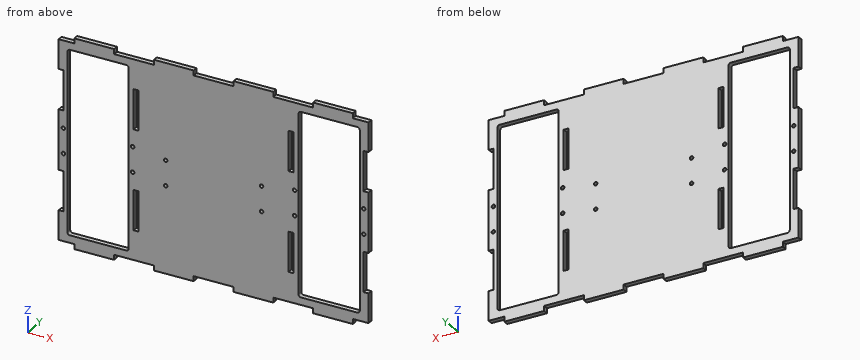
from build123d import *

# Parameters (mm, degrees)
SKETCH5_W             = 395.4
SKETCH5_H             = 265.4
BOSS_EXTRUDE3_DEPTH   = 6.35
SKETCH6_W             = 78.175
SKETCH6_H             = 243.175
SKETCH6_W_2           = 75
SKETCH6_H_2           = 240
CUT_EXTRUDE1_DEPTH    = 6.35
F_4_0MM_DOWEL_HOLE1_D = 4.5
SKETCH10_W            = 6.35
SKETCH10_H            = 50.8
SKETCH10_W_2          = 50.8
SKETCH10_H_2          = 6.35
CUT_EXTRUDE2_DEPTH    = 6.35
SKETCH11_W            = 50.8
SKETCH11_H            = 6.35
CUT_EXTRUDE3_DEPTH    = 6.35
SKETCH12_W            = 78.175
SKETCH12_H            = 4.7625
BOSS_EXTRUDE4_DEPTH   = 6.35
FILLET1_R             = 3.175


with BuildPart() as part:
    # Sketch5 → Boss-Extrude3 (new body)
    with BuildSketch(Plane(origin=(0, 0, 0), x_dir=(1, 0, 0), z_dir=(0, 1, 0))):
        Rectangle(SKETCH5_W, SKETCH5_H)
    extrude(amount=BOSS_EXTRUDE3_DEPTH)

    # Sketch6 → Cut-Extrude1 (cut)
    # profile 1 of 4: a face of its own
    with BuildSketch(Plane(origin=(0, 6.35, 0), x_dir=(1, 0, 0), z_dir=(0, 1, 0))):
        with Locations((147.5, 0)):
            Rectangle(SKETCH6_W, SKETCH6_H)
        with Locations((147.5, 0)):
            Rectangle(SKETCH6_W_2, SKETCH6_H_2, mode=Mode.SUBTRACT)
    # profile 2 of 4: a face of its own
    with BuildSketch(Plane(origin=(0, 6.35, 0), x_dir=(1, 0, 0), z_dir=(0, 1, 0))):
        with Locations((147.5, 0)):
            Rectangle(SKETCH6_W_2, SKETCH6_H_2)
    # profile 3 of 4: a face of its own
    with BuildSketch(Plane(origin=(0, 6.35, 0), x_dir=(1, 0, 0), z_dir=(0, 1, 0))):
        with Locations((-147.5, 0)):
            Rectangle(SKETCH6_W, SKETCH6_H)
        with Locations((-147.5, 0)):
            Rectangle(SKETCH6_W_2, SKETCH6_H_2, mode=Mode.SUBTRACT)
    # profile 4 of 4: a face of its own
    with BuildSketch(Plane(origin=(0, 6.35, 0), x_dir=(1, 0, 0), z_dir=(0, 1, 0))):
        with Locations((-147.5, 0)):
            Rectangle(SKETCH6_W_2, SKETCH6_H_2)
    extrude(amount=-CUT_EXTRUDE1_DEPTH, mode=Mode.SUBTRACT)

    # Ø4.0mm Dowel Hole1 (through all)
    with Locations(Plane(origin=(0, 6.35, 0), x_dir=(1, 0, 0), z_dir=(0, 1, 0))):
        with Locations((191.675, -16), (191.675, 16), (103.325, -16), (103.325, 16), (-191.675, -16), (-191.675, 16), (-103.325, -16), (-103.325, 16), (-61.175, -10), (-61.175, 22), (61.175, 22), (61.175, -10)):
            Hole(F_4_0MM_DOWEL_HOLE1_D / 2)

    # Sketch10 → Cut-Extrude2 (cut)
    with BuildSketch(Plane.XZ):
        with Locations((98.8875, -63.5)):
            Rectangle(SKETCH10_W, SKETCH10_H)
        with Locations((98.8875, 63.5)):
            Rectangle(SKETCH10_W, SKETCH10_H)
        with Locations((-98.8875, 63.5)):
            Rectangle(SKETCH10_W, SKETCH10_H)
        with Locations((-98.8875, -63.5)):
            Rectangle(SKETCH10_W, SKETCH10_H)
        Polygon((197.7, 132.7), (177.8, 132.7), (177.8, 126.35), (191.35, 126.35), (197.7, 126.35), align=None)
        Polygon((127, 132.7), (76.2, 132.7), (76.2, 126.35), (95.7125, 126.35), (102.0625, 126.35), (108.4125, 126.35), (127, 126.35), align=None)
        with Locations((0, 129.525)):
            Rectangle(SKETCH10_W_2, SKETCH10_H_2)
        Polygon((-127, 132.7), (-127, 126.35), (-108.4125, 126.35), (-102.0625, 126.35), (-95.7125, 126.35), (-76.2, 126.35), (-76.2, 132.7), align=None)
        Polygon((-197.7, 126.35), (-191.35, 126.35), (-177.8, 126.35), (-177.8, 132.7), (-197.7, 132.7), align=None)
        Polygon((-177.8, -126.35), (-191.35, -126.35), (-197.7, -126.35), (-197.7, -132.7), (-177.8, -132.7), align=None)
        Polygon((-108.4125, -126.35), (-127, -126.35), (-127, -132.7), (-76.2, -132.7), (-76.2, -126.35), (-95.7125, -126.35), (-102.0625, -126.35), align=None)
        with Locations((0, -129.525)):
            Rectangle(SKETCH10_W_2, SKETCH10_H_2)
        Polygon((76.2, -126.35), (76.2, -132.7), (127, -132.7), (127, -126.35), (108.4125, -126.35), (102.0625, -126.35), (95.7125, -126.35), align=None)
        Polygon((177.8, -126.35), (177.8, -132.7), (197.7, -132.7), (197.7, -126.35), (191.35, -126.35), align=None)
    extrude(amount=-CUT_EXTRUDE2_DEPTH, mode=Mode.SUBTRACT)

    # Sketch11 → Cut-Extrude3 (cut)
    with BuildSketch(Plane(origin=(197.7, 0, 0), x_dir=(0, 0, -1), z_dir=(1, 0, 0))):
        with Locations((-63.5, 3.175)):
            Rectangle(SKETCH11_W, SKETCH11_H)
        with Locations((63.5, 3.175)):
            Rectangle(SKETCH11_W, SKETCH11_H)
    cut_extrude3 = extrude(amount=-CUT_EXTRUDE3_DEPTH, mode=Mode.SUBTRACT)

    # Mirror1: Cut-Extrude3 across plane
    add(cut_extrude3.mirror(Plane(origin=(0, 0, 0), x_dir=(0, 0, 1), z_dir=(1, 0, 0))), mode=Mode.SUBTRACT)

    # Sketch12 → Boss-Extrude4 (add)
    with BuildSketch(Plane.XZ):
        with Locations((147.5, -119.20625)):
            Rectangle(SKETCH12_W, SKETCH12_H)
        with Locations((147.5, 119.20625)):
            Rectangle(SKETCH12_W, SKETCH12_H)
        with Locations((-147.5, 119.20625)):
            Rectangle(SKETCH12_W, SKETCH12_H)
        with Locations((-147.5, -119.20625)):
            Rectangle(SKETCH12_W, SKETCH12_H)
    extrude(amount=-BOSS_EXTRUDE4_DEPTH)

    # Fillet1
    fillet1_edges = [part.edges().sort_by_distance(p)[0] for p in [
        (108.4125, 3.175, -116.825),
        (186.5875, 3.175, -116.825),
        (186.5875, 3.175, 116.825),
        (108.4125, 3.175, 116.825),
        (-186.5875, 3.175, 116.825),
        (-108.4125, 3.175, 116.825),
        (-108.4125, 3.175, -116.825),
        (-186.5875, 3.175, -116.825),
    ]]
    fillet(fillet1_edges, radius=FILLET1_R)


solid = part.part
Work out the finished part from the listing and answer in its coordinate system (mm). Give positions to 0.01 mm unless a question says otherwise; leave off trailing zeros. Loops run counter-clockwise (first coordinate to the right, second up) from the corner with the lowest first, then second, coordinate; pieces in that order, holes last. Notation, with made-up numbers: (29, 85) -> (73, 85) arc R9 ccw to (73, 97) -> close; hole circle Ø1 at (10, -25). An arc over 180 degrees is marked (long way). Use a Markdown table: item, result. Add a question column.
1. Flat-ended cylindrical pins translate along their axes: pin 1 Ø3 at (y, z) = (2, -51) entering from +X; pin 2 Ø3 at (x, y) = (-98.5, 4.5) entering from +Z; pin 3 Ø3 at (x, y) = (195.5, 3.5) entering from -Z. Find the tip coordinate at first contact, or state that the pin passes through.
2. Section D-D on x = 2 is taken. Determine the outline of the cut face in (y, z).
3. Section C-C on y = 3.25 is taken. State how many separate pieces and enclosed holes the cut face has, and give its area (3 significant figures).
4. Section A-A on z = -64 is taken. Determine the outline of the cut face in (x, y), and give its area (3 significant figures).
5. Section B-B on x = -116.5 is taken. Determine the outline of the cut face in (y, z) (3 decimals).
6. Find the intervals of material crossed by probe 1 along X at (y, z) = (2, -22.5); probe 2 along X at (y, z) = (1.75, -69); probe 3 along X at (y, z) = (5.5, 27.5), in increasing order.
Results below:
| question | item | result |
|---|---|---|
| 1 | pin 1 | stops at x = 191.35 |
| 1 | pin 2 | stops at z = 126.35 |
| 1 | pin 3 | stops at z = -126.35 |
| 2 | outline | (0, -126.35) -> (6.35, -126.35) -> (6.35, 126.35) -> (0, 126.35) -> close |
| 3 | separate pieces | 1 |
| 3 | enclosed holes | 18 |
| 3 | area | 63,200 mm^2 |
| 4 | outline | (-191.35, 0) -> (-186.59, 0) -> (-186.59, 6.35) -> (-191.35, 6.35) -> close; (-108.41, 0) -> (-102.06, 0) -> (-102.06, 6.35) -> (-108.41, 6.35) -> close; (-95.71, 0) -> (95.71, 0) -> (95.71, 6.35) -> (-95.71, 6.35) -> close; (102.06, 0) -> (108.41, 0) -> (108.41, 6.35) -> (102.06, 6.35) -> close; (186.59, 0) -> (191.35, 0) -> (191.35, 6.35) -> (186.59, 6.35) -> close |
| 4 | area | 1,360 mm^2 |
| 5 | outline | (0, -126.35) -> (6.35, -126.35) -> (6.35, -116.825) -> (0, -116.825) -> close; (0, 116.825) -> (6.35, 116.825) -> (6.35, 126.35) -> (0, 126.35) -> close |
| 6 | probe 1 | x = -197.7 to -186.59, -108.41 to -63.37, -58.98 to 58.98, 63.37 to 108.41, 186.59 to 197.7 |
| 6 | probe 2 | x = -191.35 to -186.59, -108.41 to -102.06, -95.71 to 95.71, 102.06 to 108.41, 186.59 to 191.35 |
| 6 | probe 3 | x = -197.7 to -186.59, -108.41 to 108.41, 186.59 to 197.7 |
